Study the drawing (mm; zero at the part's minimum x, y, z) and answer. A direction names the side the tool comes from. Give positions to 0.01 mm unless a question says otherwise; leave off trailing zeros. Write each loop counter-clockwise with the first axis right and the second up, starting at its lowest first coordinate (ties: lowest second). Pieces come first, ordered by that corner, then holes. Notation, with made-up numbers: (29.25, 46.5) -> (81.25, 46.5) arc R18 ccw to (81.25, 63.5) -> close; hole circle Ø5 at (73, 75.5). An arc over 180 degrees is marked (long way). One line per question, with ' | ' between items.
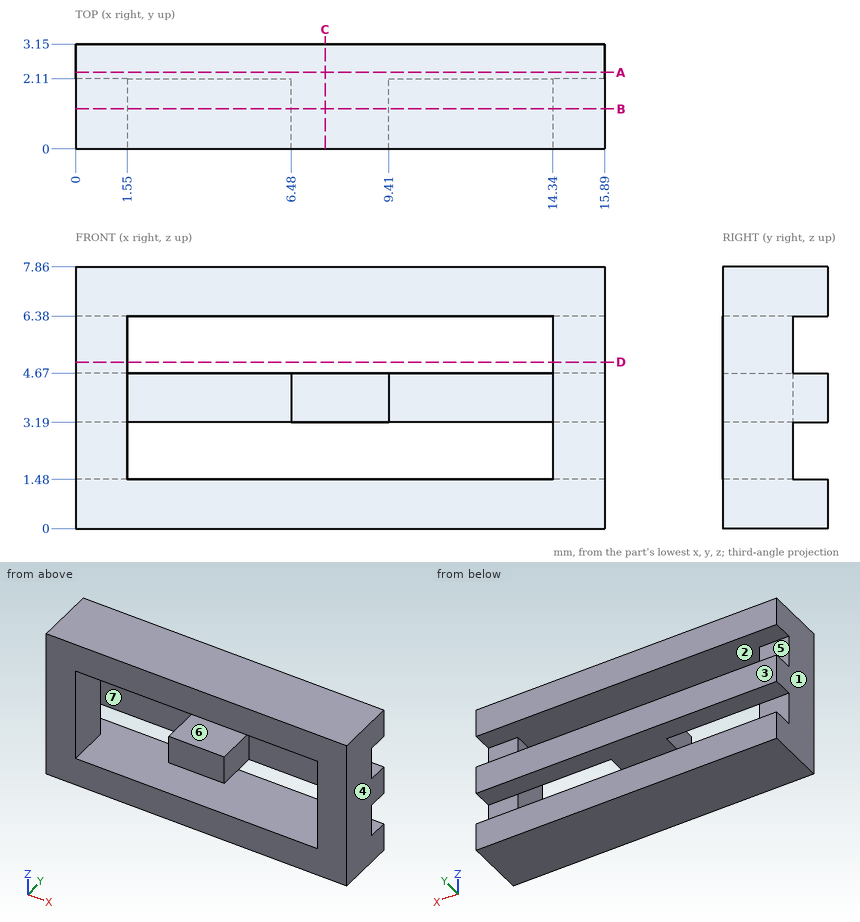
Item 1: Find section C-C (x = 7.5). Write down the section's boundary in (y, z), then the cut area to 3 significant figures.
Answers below:
outline: (0, 0) -> (3.15, 0) -> (3.15, 1.48) -> (0, 1.48) -> close; (0, 3.19) -> (3.15, 3.19) -> (3.15, 4.67) -> (0, 4.67) -> close; (0, 6.38) -> (3.15, 6.38) -> (3.15, 7.86) -> (0, 7.86) -> close | area: 14.0 mm²
Item 2: Determine the mould class of the marked faces 1, 2, 3 and 4 for opening direction X: pulls with the +X half, pulls with the -X half, needs draft (parallel to the pull), parting line crosses it, or undercut.
Answers below:
face 1: pulls with the -X half | face 2: undercut | face 3: needs draft | face 4: pulls with the +X half
Item 3: Find section B-B (y = 1.2). Write down the section's boundary in (x, z), then the cut area to 3 significant figures.
Answers below:
outline: (0, 0) -> (15.89, 0) -> (15.89, 7.86) -> (0, 7.86) -> close; (6.48, 3.19) -> (9.41, 3.19) -> (9.41, 4.67) -> (6.48, 4.67) -> close; hole (1.55, 1.48) -> (14.34, 1.48) -> (14.34, 6.38) -> (1.55, 6.38) -> close | area: 66.6 mm²
Item 4: Consider line 1 (Z direction, x = 11.25, y = 3.05); line 2 (X direction, y = 1.15, z = 2.5); line 3 (Z direction, x = 4.25, y = 0.75). Determine where each line is inside the solid, lowest interval first. Write a range as [from, to].
Answers below:
line 1: [0, 1.48], [3.19, 4.67], [6.38, 7.86] | line 2: [0, 1.55], [14.34, 15.89] | line 3: [0, 1.48], [6.38, 7.86]
Item 5: Find section D-D (z = 5). Write down the section's boundary in (x, y), then the cut area to 3 significant figures.
Answers below:
outline: (0, 0) -> (1.55, 0) -> (1.55, 2.11) -> (0, 2.11) -> close; (14.34, 0) -> (15.89, 0) -> (15.89, 2.11) -> (14.34, 2.11) -> close | area: 6.54 mm²
Item 6: A tool of negligible diameter and unlimited length cuts with its end or side. For the marked faces 5, 6 and 7, from which of +Z, -Z, +X, -X, +Y, -Y can it reach the whole face along a straight path? Write none if from no direction.
Answers below:
face 5: +X, -X, +Y | face 6: +Y | face 7: -Y
Item 7: Find section A-A (y = 2.3). Write down the section's boundary in (x, z).
Answers below:
outline: (0, 0) -> (15.89, 0) -> (15.89, 1.48) -> (0, 1.48) -> close; (0, 3.19) -> (15.89, 3.19) -> (15.89, 4.67) -> (0, 4.67) -> close; (0, 6.38) -> (15.89, 6.38) -> (15.89, 7.86) -> (0, 7.86) -> close
Item 8: Flat-ended cylindrical pins translate along their axes: pin 1 (1.2 mm diameter, centred on x = 15, z = 5.5, fed in from +Y); pin 2 (1.2 mm diameter, centred on x = 11, z = 4, fed in from -Y). Find the tip coordinate at first contact, or state that the pin passes through.
Answers below:
pin 1: y = 2.11 | pin 2: y = 2.11
